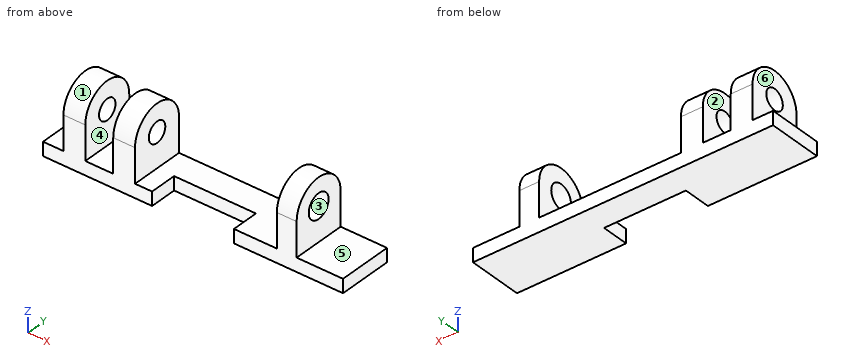
from build123d import *

# Parameters (mm, degrees)
BOSS_EXTRUDE1_START = -9.5
SKETCH1_R           = 0.75
BOSS_EXTRUDE1_DEPTH = 1.6
BOSS_EXTRUDE2_START = -5.85
SKETCH1_3_R         = 0.75
BOSS_EXTRUDE2_DEPTH = 1.6
BOSS_EXTRUDE5_START = 7.6
SKETCH1_5_R         = 2
SKETCH1_5_R_2       = 0.9
BOSS_EXTRUDE5_DEPTH = 1.45
BOSS_EXTRUDE3_START = 11
SKETCH1_4_W         = 1
SKETCH1_4_H         = 4
BOSS_EXTRUDE3_DEPTH = 22
CUT_EXTRUDE1_START  = 3
SKETCH1_6_W         = 1
SKETCH1_6_H         = 2
CUT_EXTRUDE1_DEPTH  = 6


with BuildPart() as part:
    # Sketch1 → Boss-Extrude1 (new body)
    with BuildSketch(Plane(origin=(0, 0, 0), x_dir=(0, 0, -1), z_dir=(1, 0, 0)).offset(BOSS_EXTRUDE1_START)):
        with BuildLine():
            Line((2.5, 2), (0, 2))
            ThreePointArc((0, 2), (-2, 0), (0, -2))
            Line((0, -2), (2.5, -2))
            Line((2.5, -2), (2.5, 2))
        make_face()
        with Locations(Location((0, 0, 0), (0, 0, 180))):
            Circle(SKETCH1_R, mode=Mode.SUBTRACT)
    extrude(amount=BOSS_EXTRUDE1_DEPTH)



with BuildPart() as body_2:
    # Sketch1<3> → Boss-Extrude2 (new body)
    with BuildSketch(Plane(origin=(0, 0, 0), x_dir=(0, 0, -1), z_dir=(1, 0, 0)).offset(BOSS_EXTRUDE2_START)):
        with BuildLine():
            Line((2.5, 2), (0, 2))
            ThreePointArc((0, 2), (-2, 0), (0, -2))
            Line((0, -2), (2.5, -2))
            Line((2.5, -2), (2.5, 2))
        make_face()
        with Locations(Location((0, 0, 0), (0, 0, 180))):
            Circle(SKETCH1_3_R, mode=Mode.SUBTRACT)
    extrude(amount=BOSS_EXTRUDE2_DEPTH)


with BuildPart() as body_3:
    # Sketch1<5> → Boss-Extrude5 (new body)
    with BuildSketch(Plane(origin=(0, 0, 0), x_dir=(0, 0, -1), z_dir=(1, 0, 0)).offset(BOSS_EXTRUDE5_START)):
        Circle(SKETCH1_5_R)
        Circle(SKETCH1_5_R_2, mode=Mode.SUBTRACT)
        with BuildLine():
            Line((2.5, 2), (0, 2))
            ThreePointArc((0, 2), (1.414213562, 1.414213562), (2, 0))
            ThreePointArc((2, 0), (1.414213562, -1.414213562), (0, -2))
            Line((0, -2), (2.5, -2))
            Line((2.5, -2), (2.5, 0))
            Line((2.5, 0), (2.5, 2))
        make_face()
    extrude(amount=-BOSS_EXTRUDE5_DEPTH)


with BuildPart() as part_1:
    add(part.part)

    add(body_2.part)  # Boss-Extrude3 merges body 2

    add(body_3.part)  # Boss-Extrude3 merges body 3
    # Sketch1<4> → Boss-Extrude3 (add)
    with BuildSketch(Plane(origin=(0, 0, 0), x_dir=(0, 0, -1), z_dir=(1, 0, 0)).offset(BOSS_EXTRUDE3_START)):
        with Locations((3, 0)):
            Rectangle(SKETCH1_4_W, SKETCH1_4_H)
    extrude(amount=-BOSS_EXTRUDE3_DEPTH)

    # Sketch1<6> → Cut-Extrude1 (cut)
    with BuildSketch(Plane(origin=(0, 0, 0), x_dir=(0, 0, -1), z_dir=(1, 0, 0)).offset(CUT_EXTRUDE1_START)):
        with Locations((3, -1)):
            Rectangle(SKETCH1_6_W, SKETCH1_6_H)
    extrude(amount=-CUT_EXTRUDE1_DEPTH, mode=Mode.SUBTRACT)


solid = part_1.part
Could you check a few things on this model? Use its own coordinates, in mm. Face numbers are marked on the shaded views. A direction names the side the tool comes from. Coordinates: 2 decimals unless noted, no trailing zeros. Loops run counter-clockwise (first coordinate to the right, second up) from the corner with the lowest first, then second, coordinate; pieces in that order, holes last.
1. We'd pull the mould along Z, two halves only. Please class the marked faces 1, 2 and 3: released by +Z, released by -Z, zero draft, split by the parting line, or undercut.
2. For the marked faces 4, 5 and 6, which set-ups out of +Z, -Z, +X, -X, +Y, -Y let a thin tool reach every point of the face, with its end or its side?
3. Imagine slicing it at C-C (z = 0.45). Please give me the cut outline in (x, y).
4. For P1, Ø1, axis at x = -7.5, z = 0.5, coming from the +Y side; P2, Ø1.5, axis at y = -1, z = 0.5, coming from the -X side; P3, Ø1.2, axis at x = -10, y = -0.5, coming from the +Z side, each with a flat end and sliding along its axis, tell me the tip position at first contact or that it passes through.
5. I need wall thicknesses on L1, parallel to X at y = -1.3, z = 0.95; L2, parallel to X at y = -1.55, z = -2.9; L3, parallel to Y at x = 2.25, z = -2.85. Which ranges of each line are inside material? Lowest first, please.
6. Imagine slicing it at D-D (y = -0.55). Give the number of separate pieces and of enclosed holes in the cut face, and give its area (3 significant figures).
7. Imagine slicing it at A-A (y = 0.35). Please give me the cut outline in (x, z).
8. Imagine slicing it at B-B (x = 6.5). Please give me the cut outline in (y, z).
Computed values:
1. face 1: released by +Z
1. face 2: zero draft
1. face 3: undercut
2. face 4: +Z, +Y, -Y
2. face 5: +Z, +X, +Y, -Y
2. face 6: +Z, -X, +Y, -Y
3. outline: (-9.5, -1.95) - (-7.9, -1.95) - (-7.9, -0.6) - (-9.5, -0.6) - close; (-9.5, 0.6) - (-7.9, 0.6) - (-7.9, 1.95) - (-9.5, 1.95) - close; (-5.85, -1.95) - (-4.25, -1.95) - (-4.25, -0.6) - (-5.85, -0.6) - close; (-5.85, 0.6) - (-4.25, 0.6) - (-4.25, 1.95) - (-5.85, 1.95) - close; (6.15, -1.95) - (7.6, -1.95) - (7.6, -0.78) - (6.15, -0.78) - close; (6.15, 0.78) - (7.6, 0.78) - (7.6, 1.95) - (6.15, 1.95) - close
4. P1: stops at y = 1.99
4. P2: stops at x = -9.5
4. P3: stops at z = 1.99
5. L1: x = -9.5 to -7.9, -5.85 to -4.25, 6.15 to 7.6
5. L2: x = -11 to -3, 3 to 11
5. L3: y = 0 to 2
6. separate pieces: 5
6. enclosed holes: 0
6. area: 31.2 mm2
7. outline: (-11, -3.5) - (11, -3.5) - (11, -2.5) - (7.6, -2.5) - (7.6, -0.83) - (6.15, -0.83) - (6.15, -2.5) - (-4.25, -2.5) - (-4.25, -0.66) - (-5.85, -0.66) - (-5.85, -2.5) - (-7.9, -2.5) - (-7.9, -0.66) - (-9.5, -0.66) - (-9.5, -2.5) - (-11, -2.5) - close; (-9.5, 0.66) - (-7.9, 0.66) - (-7.9, 1.97) - (-9.5, 1.97) - close; (-5.85, 0.66) - (-4.25, 0.66) - (-4.25, 1.97) - (-5.85, 1.97) - close; (6.15, 0.83) - (7.6, 0.83) - (7.6, 1.97) - (6.15, 1.97) - close
8. outline: (-2, -3.5) - (2, -3.5) - (2, 0) arc R2 ccw to (-2, 0) - close; hole circle Ø1.8 at (0, 0)
